The model under review builds one solid part; all positions refer to its coordinate system, in mm. Face numbers are marked on the shaded views. A direction names the side the tool comes from. Coordinates: 2 decimals unless noted, no trailing zeros. Write each loop counter-clockwise with the first axis right and the second up, starting at its lowest first coordinate (ties: lowest second). Pieces come first, ordered by that corner, then holes.
1) Add section B-B, the plane y = -21.5. State the section outline as (x, z) points, then the cut area to 3 significant figures.
2) Add section D-D, the plane x = 49.5. State the section outline as (y, z) points.
3) Mouldability with a two-part tool opening along Z and no side actions: class the marked faces 6, 7, 8 and 9 as released by +Z, released by -Z, zero draft, split by the parting line, or undercut.
4) For P1, Ø12.5, axis at y = 3.5, z = 2.5, coming from the -X side; P2, Ø5, axis at y = -1.5, z = 4, coming from the +X side; P3, Ø4.5, axis at x = 49, z = 2.5, coming from the +Y side, all flat-tipped, find the tip position at first contact; note any pin that passes through.
5) For line 1 (Z direction, x = 54, y = -22); line 2 (Y direction, x = 10.25, z = 7.5); line 3 (X direction, y = -21.5, z = -4), list the stretches that pass through material, from the lowest coordinate up.
6) Machinability: for the marked faces 1, 2, 3, 4 and 5, which of the approach directions +Z, -Z, +X, -X, +Y, -Y give a long, thin tool a straight path to every point of the face, cutting with its end or side? Answer none if there is none.
7) Add section C-C, the plane x = 38. State the section outline as (y, z) points, then the cut area to 3 significant figures.
8) Add section A-A, the plane x = 25. State the section outline as (y, z) points.
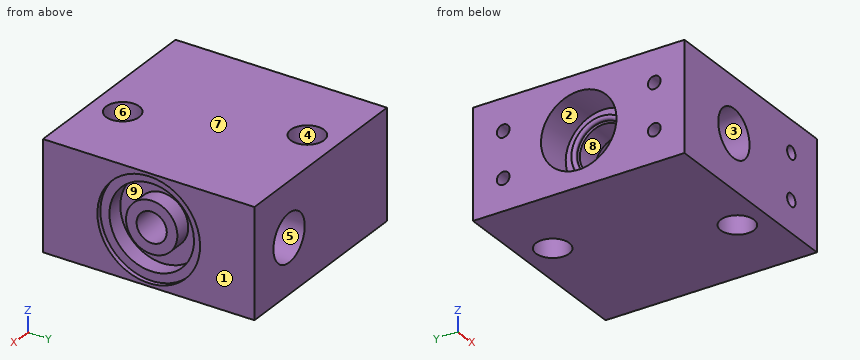
from build123d import *

# Parameters (mm, degrees)
ESQUISSE1_W                                   = 67
ESQUISSE1_H                                   = 70
BASE_EXTRUSION_DEPTH                          = 18
ESQUISSE8_R                                   = 2.851179932
ENL_V_MAT_EXTRU_1_DEPTH                       = 29
ESQUISSE9_R                                   = 5.5
TROUS_DE_PASSAGE_POUR_FIXATIONMAT_EXTRU_DEPTH = 84.725742756
R_P_TITION_LIN_AIRE1_COUNT                    = 2
R_P_TITION_LIN_AIRE1_PITCH                    = 15
R_P_TITION_LIN_AIRE1_COUNT_DIR2               = 2
R_P_TITION_LIN_AIRE1_PITCH_DIR2               = 50


with BuildPart() as part:
    # Esquisse1 → Base-Extrusion (new, symmetric)
    with BuildSketch(Plane.XY):
        with Locations((33.5, 0)):
            Rectangle(ESQUISSE1_W, ESQUISSE1_H)
    extrude(amount=BASE_EXTRUSION_DEPTH, both=True)

    # Esquisse2 → Enlèvement de matière-Révolution1 (revolve, cut)
    with BuildSketch(Plane.XY, mode=Mode.PRIVATE) as enl_vement_de_mati_re_r_volution1_sk:
        with BuildLine():
            Line((0, 12.5), (12.5, 12.5))
            Line((12.5, 12.5), (12.5, 10))
            Line((12.5, 10), (11.75, 10))
            ThreePointArc((11.75, 10), (11, 9.25), (11.75, 8.5))
            Line((11.75, 8.5), (12.25, 8.5))
            Line((12.25, 8.5), (12.75, 8))
            Line((12.75, 8), (20.5, 8))
            Line((20.5, 8), (21.5, 9))
            Line((21.5, 9), (28.5, 9))
            Line((28.5, 9), (29.5, 8))
            Line((29.5, 8), (45, 8))
            Line((45, 8), (45, 12))
            Line((45, 12), (54, 12))
            Line((54, 12), (54, 8))
            Line((54, 8), (54, 5))
            Line((54, 5), (65.5, 5))
            Line((65.5, 5), (65.5, 8.5))
            Line((65.5, 8.5), (60, 8.5))
            Line((60, 8.5), (60, 14))
            Line((60, 14), (65.5, 14))
            Line((65.5, 14), (65.5, 17))
            Line((65.5, 17), (67, 17))
            Line((67, 17), (67, 0))
            Line((67, 0), (0, 0))
            Line((0, 0), (0, 12.5))
        make_face()
    revolve(enl_vement_de_mati_re_r_volution1_sk.sketch.rotate(Axis((-4.441074665, 0, 0), (1, 0, 0)), 90), axis=Axis((-4.441074665, 0, 0), (1, 0, 0)), mode=Mode.SUBTRACT)

    # Esquisse4 → Filetage de tuyauterie ISO 7 - Rc 3/81 (revolve, cut)
    with BuildSketch(Plane(origin=(49.5, 35, 0), x_dir=(0, 0, 1), z_dir=(1, 0, 0))):
        Polygon((0, 0), (0, 26.296153426), (7.15, 22), (7.15, 20), (7.278667579, 20), (7.903, 0), align=None)
    revolve(axis=Axis((49.5, 41.35, 0), (0, -1, 0)), mode=Mode.SUBTRACT)

    # Esquisse7 → Perçage1 (revolve, cut)
    with BuildSketch(Plane(origin=(25, -35, 0), x_dir=(0, 0, -1), z_dir=(1, 0, 0))):
        Polygon((0, 0), (0, 26.296153426), (7.15, 22), (7.15, 20), (7.278667579, 20), (7.903, 0), align=None)
    revolve(axis=Axis((25, -41.35, 0), (0, 1, 0)), mode=Mode.SUBTRACT)

    # Esquisse8 → Enlèv. mat.-Extru.1 (cut)
    with BuildSketch(Plane.XZ.offset(35)):
        with Locations(Location((25, 0, 0), (0, 0, 270))):
            Circle(ESQUISSE8_R)
    extrude(amount=-ENL_V_MAT_EXTRU_1_DEPTH, mode=Mode.SUBTRACT)

    # Esquisse9 → Trous de passage pour fixationmat.-Extru.2 (cut, through all)
    with BuildSketch(Plane.XY.offset(18)):
        with Locations((25, 25)):
            Circle(ESQUISSE9_R)
        with Locations((42, -25)):
            Circle(ESQUISSE9_R)
    extrude(amount=-TROUS_DE_PASSAGE_POUR_FIXATIONMAT_EXTRU_DEPTH, mode=Mode.SUBTRACT)

    # Esquisse10 → Trou taraudé M5x0.81 (revolve, cut)
    with BuildSketch(Plane(origin=(0, 25, 7.5), x_dir=(0, 0, 1), z_dir=(0, 1, 0))):
        Polygon((0, 0), (0, 15.2618073), (2.1, 14), (2.1, 0), align=None)
    trou_taraud_m5x0_81 = revolve(axis=Axis((-6.35, 25, 7.5), (1, 0, 0)), mode=Mode.SUBTRACT)

    # Répétition linéaire1: Trou taraud_ M5x0.81 2 × 2
    with Locations(*[(0, -j * R_P_TITION_LIN_AIRE1_PITCH_DIR2, -i * R_P_TITION_LIN_AIRE1_PITCH) for i in range(R_P_TITION_LIN_AIRE1_COUNT) for j in range(R_P_TITION_LIN_AIRE1_COUNT_DIR2) if (i, j) != (0, 0)]):
        add(trou_taraud_m5x0_81, mode=Mode.SUBTRACT)

    # Esquisse12 → Trou taraudé M5x0.82 (revolve, cut)
    with BuildSketch(Plane(origin=(54, -35, -7.5), x_dir=(0, 0, -1), z_dir=(1, 0, 0))):
        Polygon((0, 0), (0, 19.2618073), (2.1, 18), (2.1, 0), align=None)
    trou_taraud_m5x0_82 = revolve(axis=Axis((54, -41.35, -7.5), (0, 1, 0)), mode=Mode.SUBTRACT)

    # Symétrie1: Trou taraudé M5x0.82 across plane
    add(trou_taraud_m5x0_82.mirror(Plane.XY), mode=Mode.SUBTRACT)


solid = part.part
Geometry results:
1. outline: (0, -18) - (37.76, -18) - (37.76, 18) - (0, 18) - close; (46.24, -18) - (67, -18) - (67, 18) - (46.24, 18) - close; hole circle Ø14.96 at (25, 0); hole circle Ø4.2 at (54, -7.5); hole circle Ø4.2 at (54, 7.5)
1. area: 1,900 mm2
2. outline: (-35, -18) - (35, -18) - (35, -7.9) - (15, -7.28) - (15, -7.15) - (13, -7.15) - (11.24, -4.21) arc R12 cw (long way) to (11.24, 4.21) - (13, 7.15) - (15, 7.15) - (15, 7.28) - (35, 7.9) - (35, 18) - (-35, 18) - close
3. face 6: zero draft
3. face 7: released by +Z
3. face 8: undercut
3. face 9: undercut
4. P1: stops at x = 11
4. P2: stops at x = 65.5
4. P3: stops at y = 11.59
5. line 1: z = -18 to -9.6, -5.4 to 5.4, 9.6 to 18
5. line 2: y = -35 to -27.1, -22.9 to -10, 10 to 22.9, 27.1 to 35
5. line 3: x = 0 to 18.68, 31.32 to 37.76, 46.24 to 67
6. face 1: +Z, -Z, +X, +Y, -Y
6. face 2: -X
6. face 3: -Y
6. face 4: +Z, -Z
6. face 5: +Y
7. outline: (-35, -18) - (-28.77, -18) - (-28.77, 18) - (-35, 18) - close; (-21.23, -18) - (35, -18) - (35, 18) - (-21.23, 18) - close; hole circle Ø16 at (0, 0)
7. area: 2,050 mm2
8. outline: (-35, -18) - (19.5, -18) - (19.5, 18) - (-35, 18) - (-35, 7.9) - (-15, 7.28) - (-15, 7.15) - (-13, 7.15) - (-10.42, 2.85) - (-8.54, 2.85) arc R9 cw (long way) to (-8.54, -2.85) - (-10.42, -2.85) - (-13, -7.15) - (-15, -7.15) - (-15, -7.28) - (-35, -7.9) - close; (30.5, -18) - (35, -18) - (35, 18) - (30.5, 18) - close
